```python
from build123d import *

# Parameters (mm, degrees)
SKETCH_1_W          = 7.5
SKETCH_1_H          = 9.347826087
SKETCH_1_H_2        = 10
EXTRUDE_1_DEPTH     = 3
SKETCH_2_R          = 2.2
CUT_EXTRUDE_1_DEPTH = 4
M3X0_5_1_D          = 2.5
M3X0_5_1_DEPTH      = 8.5
M3X0_5_1_TIP        = 0.751075774
SKETCH_6_W          = 69
SKETCH_6_H          = 3
CUT_EXTRUDE_2_DEPTH = 20
SKETCH_7_W          = 69
SKETCH_7_H          = 3
EXTRUDE_2_DEPTH     = 10
M3X0_5_2_D          = 2.5
M3X0_5_2_DEPTH      = 8.5
M3X0_5_2_TIP        = 0.751075774


with BuildPart() as part:
    # ｽｹｯﾁ1 → ﾎﾞｽ - 押し出し1 (new body)
    with BuildSketch(Plane.XY):
        Polygon((27, 43), (-27, 43), (-27, 33.652173913), (-34.5, 33.652173913), (-34.5, -33), (-27, -33), (-27, -43), (27, -43), (27, -33), (34.5, -33), (34.5, 33.652173913), (27, 33.652173913), align=None)
        with Locations((-30.75, 38.326086956)):
            Rectangle(SKETCH_1_W, SKETCH_1_H)
        with Locations((30.75, 38.326086956)):
            Rectangle(SKETCH_1_W, SKETCH_1_H)
        with Locations((30.75, -38)):
            Rectangle(SKETCH_1_W, SKETCH_1_H_2)
        with Locations((-30.75, -38)):
            Rectangle(SKETCH_1_W, SKETCH_1_H_2)
    extrude(amount=EXTRUDE_1_DEPTH)

    # ｽｹｯﾁ2 → ｶｯﾄ - 押し出し1 (cut, through all)
    with BuildSketch(Plane.XY.offset(3)):
        with Locations((-27, 18)):
            Circle(SKETCH_2_R)
        with Locations((27, 18)):
            Circle(SKETCH_2_R)
        with Locations((27, -13)):
            Circle(SKETCH_2_R)
        with Locations((-27, -13)):
            Circle(SKETCH_2_R)
    extrude(amount=-CUT_EXTRUDE_1_DEPTH, mode=Mode.SUBTRACT)

    # M3x0.5 ねじ穴1
    with Locations(Plane(origin=(-15.5, 24, 3), x_dir=(1, 0, 0), z_dir=(0, 0, 1))):
        with Locations((0, 0), (31, 0), (0, 16), (31, 16)):
            Hole(M3X0_5_1_D / 2, depth=M3X0_5_1_DEPTH)
            with Locations((0, 0, -(M3X0_5_1_DEPTH + M3X0_5_1_TIP / 2))):  # 118° drill point
                Cone(0, M3X0_5_1_D / 2, M3X0_5_1_TIP, mode=Mode.SUBTRACT)

    # ｽｹｯﾁ6 → ｶｯﾄ - 押し出し2 (cut)
    with BuildSketch(Plane(origin=(0, -43, 0), x_dir=(-1, 0, 0), z_dir=(0, -1, 0))):
        with Locations((0, -1.5)):
            Rectangle(SKETCH_6_W, SKETCH_6_H)
    extrude(amount=-CUT_EXTRUDE_2_DEPTH, mode=Mode.SUBTRACT)

    # ｽｹｯﾁ7 → ﾎﾞｽ - 押し出し2 (add)
    with BuildSketch(Plane(origin=(0, -23, 0), x_dir=(-1, 0, 0), z_dir=(0, -1, 0))):
        with Locations((0, -1.5)):
            Rectangle(SKETCH_7_W, SKETCH_7_H)
    extrude(amount=EXTRUDE_2_DEPTH)

    # M3x0.5 ねじ穴2
    with Locations(Plane(origin=(0, -19.574626956, 3), x_dir=(1, 0, 0), z_dir=(0, 0, 1))):
        with Locations((0, 0), (22.2, -10.3)):
            Hole(M3X0_5_2_D / 2, depth=M3X0_5_2_DEPTH)
            with Locations((0, 0, -(M3X0_5_2_DEPTH + M3X0_5_2_TIP / 2))):  # 118° drill point
                Cone(0, M3X0_5_2_D / 2, M3X0_5_2_TIP, mode=Mode.SUBTRACT)


solid = part.part
```
Build history of the part. All positions in model axes, mm. Give positions to 0.01 mm unless a question says otherwise; leave off trailing zeros. Order: outer loops, then holes, each group sorted by start corner. A loop starts at its lowest first (then second) coordinate and runs counter-clockwise, first axis right, second up. Notation, with made-up numbers: M 29.5,78.5 L 34.5,78.5 A20 ccw 34.5,92.5 Z; hole C 0.5,-28.5 d10. An arc over 180 degrees is marked long. Write item = value, one per line. Start each with the question number.
(1) Probe L1, parallel to Y at x = 27, z = 1.15; L2, parallel to Y at x = 22.2, z = 1; L3, parallel to Y at x = -28, z = 1.65. List the from-to ranges inside material, lowest first. Write a range as [from, to].
(2) Pin check, flat tip, straight feed: pin 1 Ø2.5 at (x, y) = (27, 18) entering from +Z. Stop position of the tip, or through.
(3) Slice it at C-C on x = 0. Write the cut outline in (y, z), plus the area to 4 significant figures.
(4) Two-plate mould, pull along X, no slides. Class faces 1 (the flat face through (0, 6, 0)), 2 (the flat face through (34.5, 6, 2)), 3 (the cylindrical face through (16.75, 40.05, 1.48)): released by +X, released by -X, zero draft, split by the parting line, or undercut.
(5) Slice it at B-B on y = 18. Write the cut outline in (x, z).
(6) Slice it at A-A on x = -27. Write the cut outline in (y, z), plus the area to 3 significant figures.
(7) Slice it at D-D on z = 1.5. State how many separate pieces and enclosed holes the cut face has, plus the area to 3 significant figures.
Responses:
q1.L1 = [-33, -15.2], [-10.8, 15.8], [20.2, 43]
q1.L2 = [-33, -31.12], [-28.62, 43]
q1.L3 = [-33, -14.96], [-11.04, 16.04], [19.96, 43]
q2.pin_1 = through
q3.outline = M -33,0 L -20.82,0 L -20.82,3 L -33,3 Z; M -18.32,0 L 43,0 L 43,3 L -18.32,3 Z
q3.area = 220.5 mm2
q4.face_1 = zero draft
q4.face_2 = released by +X
q4.face_3 = undercut
q5.outline = M -34.5,0 L -29.2,0 L -29.2,3 L -34.5,3 Z; M -24.8,0 L 24.8,0 L 24.8,3 L -24.8,3 Z; M 29.2,0 L 34.5,0 L 34.5,3 L 29.2,3 Z
q6.outline = M -33,0 L -15.2,0 L -15.2,3 L -33,3 Z; M -10.8,0 L 15.8,0 L 15.8,3 L -10.8,3 Z; M 20.2,0 L 43,0 L 43,3 L 20.2,3 Z
q6.area = 202 mm2
q7.separate_pieces = 1
q7.enclosed_holes = 10
q7.area = 5,150 mm2
